Read the model definition and answer for the solid it produces. Units are mm, in the model's axes. Face numbers are marked on the shaded views. A direction names the side the tool comes from. Round coordinates to 2 decimals unless told otherwise and drop trailing zeros. Order: outer loops, then holes, each group sorted by start corner. A loop starts at its lowest first (then second) coordinate and runs counter-clockwise, first axis right, second up.
from build123d import *

# Parameters (mm, degrees)
SKETCH_1_R          = 31.5
EXTRUDE_1_DEPTH     = 7.5
SKETCH_2_R          = 15.75
EXTRUDE_2_DEPTH     = 2.5
CHAMFER_1_SIZE      = 1
CHAMFER_2_SIZE      = 1
SKETCH_3_R          = 3.25
SKETCH_3_R_2        = 3
CUT_EXTRUDE_1_DEPTH = 6.5
SKETCH_4_R          = 5.5
CUT_EXTRUDE_2_DEPTH = 4
SKETCH_9_R          = 15.75
EXTRUDE_5_DEPTH     = 5
SKETCH_10_W         = 1.475
SKETCH_10_H         = 34.619836182
SKETCH_12_W         = 34.390944704
SKETCH_12_H         = 1.475


with BuildPart() as part:
    # 草图1 → 凸台-拉伸1 (new body)
    with BuildSketch(Plane.XY):
        Circle(SKETCH_1_R)
    extrude(amount=EXTRUDE_1_DEPTH)

    # 草图2 → 凸台-拉伸2 (add)
    with BuildSketch(Plane.XY.offset(7.5)):
        Circle(SKETCH_2_R)
    extrude(amount=EXTRUDE_2_DEPTH)

    # 倒角1
    chamfer_1_edges = [part.edges().sort_by_distance(p)[0] for p in [
        (-15.75, 0, 10),
    ]]
    chamfer(chamfer_1_edges, length=CHAMFER_1_SIZE)

    # 倒角2
    chamfer_2_edges = [part.edges().sort_by_distance(p)[0] for p in [
        (-31.5, 0, 7.5),
    ]]
    chamfer(chamfer_2_edges, length=CHAMFER_2_SIZE)

    # 草图3 → 切除-拉伸1 (cut)
    with BuildSketch(Plane.XY.offset(7.5)):
        with Locations((0, 25)):
            Circle(SKETCH_3_R)
        with Locations((0, -25)):
            Circle(SKETCH_3_R)
        with Locations((-17.67766953, -17.67766953)):
            Circle(SKETCH_3_R_2)
    extrude(amount=-CUT_EXTRUDE_1_DEPTH, mode=Mode.SUBTRACT)

    # 草图4 → 切除-拉伸2 (cut)
    with BuildSketch(Plane(origin=(0, 0, 0), x_dir=(-1, 0, 0), z_dir=(0, 0, -1))):
        with Locations((0, -25)):
            Circle(SKETCH_4_R)
        with Locations((0, 25)):
            Circle(SKETCH_4_R)
    extrude(amount=-CUT_EXTRUDE_2_DEPTH, mode=Mode.SUBTRACT)

    # 草图9 → 凸台-拉伸5 (add)
    with BuildSketch(Plane(origin=(0, 0, 0), x_dir=(-1, 0, 0), z_dir=(0, 0, -1))):
        Circle(SKETCH_9_R)
    extrude(amount=EXTRUDE_5_DEPTH)

    # 草图10 → 切除-旋转1 (revolve, cut)
    with BuildSketch(Plane(origin=(0, 0, -2.5), x_dir=(-1, 0, 0), z_dir=(0, 0, -1))):
        with Locations((0.7375, 0.028611435)):
            Rectangle(SKETCH_10_W, SKETCH_10_H)
    revolve(axis=Axis((0, 17.338529526, -2.5), (0, -1, 0)), mode=Mode.SUBTRACT)

    # 草图12 → 切除-旋转2 (revolve, cut)
    with BuildSketch(Plane(origin=(0, 0, -2.5), x_dir=(-1, 0, 0), z_dir=(0, 0, -1))):
        with Locations((-0.028611435, 0.7375)):
            Rectangle(SKETCH_12_W, SKETCH_12_H)
    revolve(axis=Axis((17.224083787, 0, -2.5), (-1, 0, 0)), mode=Mode.SUBTRACT)


solid = part.part
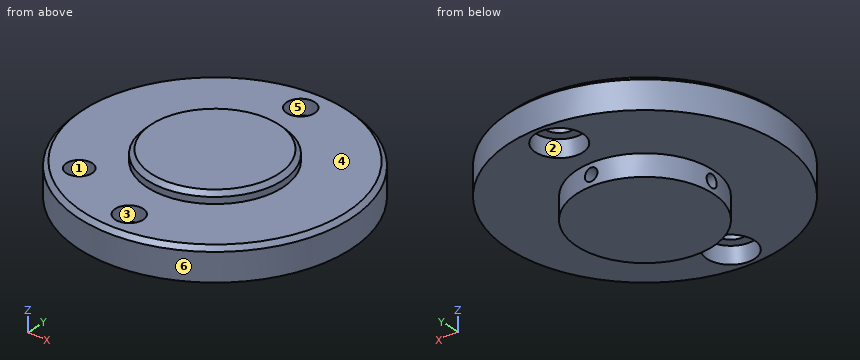
Q1. A cutting plane is placed at A-A, the plane z = -1.75. Give the vertices of the cut face in (x, y), plus the area to 3 significant figures.
Outcome:
outline: (-15.7, -1.27) arc R15.75 ccw to (-1.27, -15.7) - (-1.27, -1.27) - close; (-15.7, 1.27) - (-1.27, 1.27) - (-1.27, 15.7) arc R15.75 ccw to start; (1.27, -15.7) arc R15.75 ccw to (15.7, -1.27) - (1.27, -1.27) - close; (1.27, 1.27) - (15.7, 1.27) arc R15.75 ccw to (1.27, 15.7) - close
area: 626 mm2
Q2. For a pull along Y with two mould halves and no side action, classify the marked faces 4, 5 and 6 as released by +Y, released by -Y, zero draft, split by the parting line, or undercut.
Outcome:
face 4: zero draft
face 5: undercut
face 6: split by the parting line
Q3. For the marked faces 1, 2 and 3, determine the directions among +Z, -Z, +X, -X, +Y, -Y from which every point of the face is accessible in a straight line to the end or side of a thin tool.
Outcome:
face 1: +Z
face 2: -Z
face 3: +Z, -Z
Q4. Flat-ended cylindrical pins translate along their axes: pin 1 (12 mm diameter, centred on x = 0, y = 25, fed in from -Z); pin 2 (9 mm diameter, centred on x = 0, y = 25, fed in from -Z); pin 3 (1 mm diameter, centred on y = -14, z = 6, fed in from -X). Find the tip coordinate at first contact, or state that the pin passes through.
Outcome:
pin 1: stops at z = 0
pin 2: stops at z = 4
pin 3: stops at x = -28.46
Q5. Straight lines are drawn through the part: probe 1 along Z at (x, y) = (0, 11) (3 decimals); probe 2 along X at (y, z) = (1, 1.5); probe 3 along Z at (x, y) = (-21, 0.5). For each, find the intervals that lie inside material, in ascending order.
Outcome:
probe 1: z = -5 to -3.975, -1.025 to 10
probe 2: x = -31.48 to 31.48
probe 3: z = 0 to 7.5
